Read the model definition and answer for the solid it produces. Units are mm, in the model's axes. Coordinates: 2 decimals unless noted, no trailing zeros. Loops run counter-clockwise (first coordinate to the right, second up) from the corner with the lowest first, then second, coordinate; pieces in that order, holes last. Notation, with made-up numbers: (65.25, 67) -> (100.25, 67) arc R20 ccw to (100.25, 105) -> close; hole circle Ø2 at (62, 70.25). An arc over 180 degrees is marked (long way). Answer as a JSON object with one key per item and string values. Group by question number.
Q1. The part is cut by section A-A on y = 60.5. Write down the section's boundary in (x, z).
Q2. The part is cut by section B-B on y = 112.5. Write down the section's boundary in (x, z).
Q3. Straight lines are drawn through the part: line 1 along X through (y, z) = (3.15, 2.5); line 2 along Z through (x, y) = (10, 3.7); line 3 along Y through (x, z) = (3.25, 9). For each, find the intervals that lie inside material, in ascending order. Write a range as [from, to].
Q4. Each of these flat-tipped pins is pushed along its axis until it touches: P1, Ø10.5, axis at x = -12.5, y = 238, coming from the +Z side; P2, Ø7, axis at y = 108, z = -0.5, coming from the -X side; P3, Ø7, axis at y = 113.5, z = 1.5, coming from the +X side. Where does it stop, or does it pass through?
from build123d import *

# Parameters (mm, degrees)
SKETCH_1_W      = 30
SKETCH_1_H      = 20
SKETCH_1_R      = 1.75
EXTRUDE_1_DEPTH = 6
SKETCH_2_W      = 3
SKETCH_2_H      = 310
EXTRUDE_2_DEPTH = 30
EXTRUDE_3_DEPTH = 2.5
FILLET_1_R      = 3


with BuildPart() as part:
    # 草图1 → 凸台-拉伸1 (new body)
    with BuildSketch(Plane(origin=(0, 0, 0), x_dir=(1, 0, 0), z_dir=(0, 1, 0))):
        Rectangle(SKETCH_1_W, SKETCH_1_H)
        with Locations(Location((-10, -2.5, 0), (0, 0, 270))):
            Circle(SKETCH_1_R, mode=Mode.SUBTRACT)
        with Locations(Location((10, -2.5, 0), (0, 0, 90))):
            Circle(SKETCH_1_R, mode=Mode.SUBTRACT)
    extrude(amount=EXTRUDE_1_DEPTH)

    # 草图2 → 凸台-拉伸2 (add)
    with BuildSketch(Plane(origin=(15, 0, 0), x_dir=(0, 0, -1), z_dir=(1, 0, 0))):
        with Locations((8.5, 161)):
            Rectangle(SKETCH_2_W, SKETCH_2_H)
    extrude(amount=-EXTRUDE_2_DEPTH)

    # 草图3 → 凸台-拉伸3 (add, symmetric)
    with BuildSketch(Plane(origin=(0, 0, 0), x_dir=(0, 0, -1), z_dir=(1, 0, 0))):
        Polygon((7, 316), (-10, 6), (7, 6), align=None)
    extrude(amount=EXTRUDE_3_DEPTH, both=True)

    # 圆角1
    # the kernel refuses this fillet: 3 mm, written as the material it adds along each edge
    with BuildSketch(Plane(origin=(-5.5, 9, -4), x_dir=(0, -1, 0), z_dir=(0, 0, -1))) as fillet_1_piece_1_section:
        Polygon((0, 0), (FILLET_1_R, 0), (FILLET_1_R, -FILLET_1_R), (0, -FILLET_1_R), align=None)
    fillet_1_piece_1 = extrude(amount=FILLET_1_R, mode=Mode.PRIVATE)
    fillet_1_piece_1 = fillet_1_piece_1 - Plane(origin=(-5.5, 9, -4), x_dir=(-0.7071067811865475, 0.7071067811865475, 0), z_dir=(0, 0, -1)) * Sphere(FILLET_1_R, mode=Mode.PRIVATE)
    add(fillet_1_piece_1)
    with BuildSketch(Plane(origin=(5.5, 9, -4), x_dir=(0, -1, 0), z_dir=(0, 0, -1))) as fillet_1_piece_2_section:
        Polygon((0, 0), (FILLET_1_R, 0), (FILLET_1_R, FILLET_1_R), (0, FILLET_1_R), align=None)
    fillet_1_piece_2 = extrude(amount=FILLET_1_R, mode=Mode.PRIVATE)
    fillet_1_piece_2 = fillet_1_piece_2 - Plane(origin=(5.5, 9, -4), x_dir=(0.7071067811865475, 0.7071067811865475, 0), z_dir=(0, 0, -1)) * Sphere(FILLET_1_R, mode=Mode.PRIVATE)
    add(fillet_1_piece_2)
    with BuildSketch(Plane(origin=(-5.5, 6, -7), x_dir=(0, 0, 1), z_dir=(-1, 0, 0)), Plane(origin=(15, 6, -7), x_dir=(0, 0, 1), z_dir=(-1, 0, 0))) as fillet_1_piece_3:
        with BuildLine():
            CenterArc((FILLET_1_R, FILLET_1_R), FILLET_1_R, 180, 90)
            Line((0, FILLET_1_R), (0, 0))
            Line((0, 0), (FILLET_1_R, 0))
        make_face()
    extrude(amount=9.5)
    with BuildSketch(Plane(origin=(-2.5, 9, -7), x_dir=(-1, 0, 0), z_dir=(0, 1, 0))) as fillet_1_piece_4_section:
        with BuildLine():
            CenterArc((FILLET_1_R, FILLET_1_R), FILLET_1_R, 180, 90)
            Line((0, FILLET_1_R), (0, 0))
            Line((0, 0), (FILLET_1_R, 0))
        make_face()
    fillet_1_piece_4 = extrude(amount=307, mode=Mode.PRIVATE)
    fillet_1_piece_4 = split(fillet_1_piece_4, bisect_by=Plane(origin=(-3.194365112, 156.962181191, 1.721428773), z_dir=(0, -0.054756437403794746, -0.9984997408927277)), keep=Keep.TOP, mode=Mode.PRIVATE)
    add(fillet_1_piece_4)
    with BuildSketch(Plane(origin=(-2.5, 6, 10), x_dir=(-1, 0, 0), z_dir=(0, 0, -1))) as fillet_1_piece_5_section:
        with BuildLine():
            CenterArc((FILLET_1_R, FILLET_1_R), FILLET_1_R, 180, 90)
            Line((0, FILLET_1_R), (0, 0))
            Line((0, 0), (FILLET_1_R, 0))
        make_face()
    fillet_1_piece_5 = extrude(amount=14, mode=Mode.PRIVATE)
    fillet_1_piece_5 = split(fillet_1_piece_5, bisect_by=Plane(origin=(-3.180148424, 7.059257164, 9.941911704), z_dir=(0, -0.054756437403794746, -0.9984997408927277)), keep=Keep.TOP, mode=Mode.PRIVATE)
    add(fillet_1_piece_5)
    with BuildSketch(Plane(origin=(2.5, 9, -7), x_dir=(1, 0, 0), z_dir=(0, 1, 0))) as fillet_1_piece_6_section:
        with BuildLine():
            CenterArc((FILLET_1_R, -FILLET_1_R), FILLET_1_R, 90, 90)
            Line((0, -FILLET_1_R), (0, 0))
            Line((0, 0), (FILLET_1_R, 0))
        make_face()
    fillet_1_piece_6 = extrude(amount=307, mode=Mode.PRIVATE)
    fillet_1_piece_6 = split(fillet_1_piece_6, bisect_by=Plane(origin=(3.194365112, 156.962181191, 1.721428773), z_dir=(0, -0.054756437403794746, -0.9984997408927277)), keep=Keep.TOP, mode=Mode.PRIVATE)
    add(fillet_1_piece_6)
    with BuildSketch(Plane(origin=(2.5, 6, 10), x_dir=(1, 0, 0), z_dir=(0, 0, -1))) as fillet_1_piece_7_section:
        with BuildLine():
            CenterArc((FILLET_1_R, -FILLET_1_R), FILLET_1_R, 90, 90)
            Line((0, -FILLET_1_R), (0, 0))
            Line((0, 0), (FILLET_1_R, 0))
        make_face()
    fillet_1_piece_7 = extrude(amount=14, mode=Mode.PRIVATE)
    fillet_1_piece_7 = split(fillet_1_piece_7, bisect_by=Plane(origin=(3.180148424, 7.059257164, 9.941911704), z_dir=(0, -0.054756437403794746, -0.9984997408927277)), keep=Keep.TOP, mode=Mode.PRIVATE)
    add(fillet_1_piece_7)
    # the kernel refuses this fillet: 3 mm, written as the material it takes off along each edge
    with BuildSketch(Plane(origin=(-15, 316, 0.5), x_dir=(1, 0, 0), z_dir=(0, 0, -1))) as fillet_1_2_piece_1:
        with BuildLine():
            CenterArc((FILLET_1_R, FILLET_1_R), FILLET_1_R, 180, 90)
            Line((0, FILLET_1_R), (0, 0))
            Line((0, 0), (FILLET_1_R, 0))
        make_face()
    extrude(amount=18, mode=Mode.SUBTRACT)
    with BuildSketch(Plane(origin=(15, 316, 0.5), x_dir=(-1, 0, 0), z_dir=(0, 0, -1))) as fillet_1_2_piece_2:
        with BuildLine():
            CenterArc((FILLET_1_R, -FILLET_1_R), FILLET_1_R, 90, 90)
            Line((0, -FILLET_1_R), (0, 0))
            Line((0, 0), (FILLET_1_R, 0))
        make_face()
    extrude(amount=18, mode=Mode.SUBTRACT)
    with BuildSketch(Plane(origin=(15, -7.5, 10), x_dir=(-1, 0, 0), z_dir=(0, 1, 0))) as fillet_1_2_piece_3:
        with BuildLine():
            CenterArc((FILLET_1_R, -FILLET_1_R), FILLET_1_R, 90, 90)
            Line((0, -FILLET_1_R), (0, 0))
            Line((0, 0), (FILLET_1_R, 0))
        make_face()
    extrude(amount=21, mode=Mode.SUBTRACT)
    with BuildSketch(Plane(origin=(-15, -7.5, 10), x_dir=(1, 0, 0), z_dir=(0, 1, 0))) as fillet_1_2_piece_4:
        with BuildLine():
            CenterArc((FILLET_1_R, FILLET_1_R), FILLET_1_R, 180, 90)
            Line((0, FILLET_1_R), (0, 0))
            Line((0, 0), (FILLET_1_R, 0))
        make_face()
    extrude(amount=21, mode=Mode.SUBTRACT)


solid = part.part
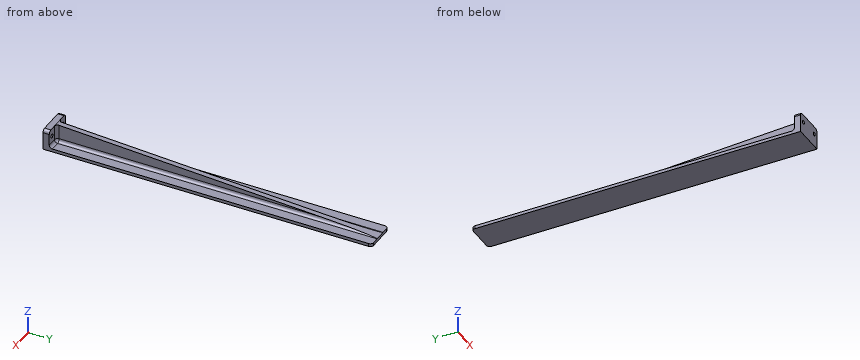
Final values:
{
 "1": {"outline": "(-15, -10) -> (15, -10) -> (15, -7) -> (5.5, -7) arc R3 cw to (2.5, -4) -> (2.5, 7.01) -> (-2.5, 7.01) -> (-2.5, -4) arc R3 cw to (-5.5, -7) -> (-15, -7) -> close"},
 "2": {"outline": "(-15, -10) -> (15, -10) -> (15, -7) -> (5.5, -7) arc R3 cw to (2.5, -4) -> (2.5, 4.16) -> (-2.5, 4.16) -> (-2.5, -4) arc R3 cw to (-5.5, -7) -> (-15, -7) -> close"},
 "3": {"line 1": "x = [-15, -11.75], [-8.25, 8.25], [11.75, 15]", "line 2": "z = [-10, 0.75], [4.25, 10]", "line 3": "y = [0, 7.02]"},
 "4": {"P1": "stops at z = -7", "P2": "stops at x = -2.5", "P3": "stops at x = 2.5"}
}
